from build123d import *

# Parameters (mm, degrees)
SKETCH1_W           = 50.8
SKETCH1_H           = 171.45
BOSS_EXTRUDE2_DEPTH = 3.175
SKETCH2_R           = 3.175
CUT_EXTRUDE1_DEPTH  = 179.84580824


with BuildPart() as part:
    # Sketch1 → Boss-Extrude2 (new body)
    with BuildSketch(Plane.XY):
        with Locations((-25.4, 85.725)):
            Rectangle(SKETCH1_W, SKETCH1_H)
    extrude(amount=-BOSS_EXTRUDE2_DEPTH)

    # Sketch2 → Cut-Extrude1 (cut, through all)
    with BuildSketch(Plane.XY):
        with Locations((-10.795, 158.75)):
            Circle(SKETCH2_R)
        with Locations((-36.83, 158.75)):
            Circle(SKETCH2_R)
        with Locations((-10.795, 133.35)):
            Circle(SKETCH2_R)
        with Locations((-36.83, 133.35)):
            Circle(SKETCH2_R)
    extrude(amount=-CUT_EXTRUDE1_DEPTH, mode=Mode.SUBTRACT)


solid = part.part
Source: CAD feature listing. Evaluate the final solid. Frame: model axes, mm. Give positions to 0.01 mm unless a question says otherwise; leave off trailing zeros. Write each loop counter-clockwise with the first axis right and the second up, starting at its lowest first coordinate (ties: lowest second). Pieces come first, ordered by that corner, then holes. Notation, with made-up numbers: (-21.75, -15) -> (23.25, -15) arc R20 ccw to (23.25, -7) -> close; hole circle Ø8 at (21, 16.5). An arc over 180 degrees is marked (long way). Return JSON: item names as keys, results as strings. Group by question number.
1. Material intervals for line 1 (X direction, y = 133.35, z = -2.25) (3 decimals); line 2 (Y direction, x = -36.83, z = -1.25) (3 decimals); line 3 (X direction, y = 160, z = -2.3), sorted ascending. Write a range as from..to.
2. Pin query (flat end, axial travel): pin 1 Ø5.5 at (x, y) = (-36.83, 133.35) entering from +Z. Return the tip coordinate at first contact, or that it passes through.
3. Section B-B, the plane y = 133.35. Output: boundary loops of the cut face in (x, z) (3 decimals), then the cut area to 3 significant figures.
4. Mould query, pull axis Y, two halves, no side actions, for faces 1 (the face through (-50.8, 85, -2)), 2 (the face through (-37.52, 130.25, -1.57)), 3 (the face through (-11.2, 161.9, -1.6)), 4 (the face through (-26, 171.45, -2)). Classes: +Y half, -Y half, draft (parallel to the pull), parting line (faces both ways), or undercut.
5. Section A-A, the plane x = -36.83. Output: boundary loops of the cut face in (y, z) (3 decimals), then the cut area to 3 significant figures.
Determined:
{
 "1": {"line 1": "x = -50.8..-40.005, -33.655..-13.97, -7.62..0", "line 2": "y = 0..130.175, 136.525..155.575, 161.925..171.45", "line 3": "x = -50.8..-39.75, -33.91..-13.71, -7.88..0"},
 "2": {"pin 1": "passes through"},
 "3": {"outline": "(-50.8, -3.175) -> (-40.005, -3.175) -> (-40.005, 0) -> (-50.8, 0) -> close; (-33.655, -3.175) -> (-13.97, -3.175) -> (-13.97, 0) -> (-33.655, 0) -> close; (-7.62, -3.175) -> (0, -3.175) -> (0, 0) -> (-7.62, 0) -> close", "area": "121 mm2"},
 "4": {"face 1": "draft", "face 2": "undercut", "face 3": "undercut", "face 4": "+Y half"},
 "5": {"outline": "(0, -3.175) -> (130.175, -3.175) -> (130.175, 0) -> (0, 0) -> close; (136.525, -3.175) -> (155.575, -3.175) -> (155.575, 0) -> (136.525, 0) -> close; (161.925, -3.175) -> (171.45, -3.175) -> (171.45, 0) -> (161.925, 0) -> close", "area": "504 mm2"}
}
